Design review of the part built by this model. Coordinates are the model's own, in mm. A direction names the side the tool comes from. Coordinates: 2 decimals unless noted, no trailing zeros. Write each loop counter-clockwise with the first axis right and the second up, starting at its lowest first coordinate (ties: lowest second). Pieces come first, ordered by that corner, then holes. Notation, with made-up numbers: M 71,41.25 L 76,41.25 A21 cw 76,59.25 Z; hole C 17.25,41.25 d10. An arc over 180 degrees is marked long. One line per question, with ' | ' between items.
from build123d import *

# Parameters (mm, degrees)
F0_W     = 165.1
F0_H     = 44.45
F1_DEPTH = 88.9
F2_W     = 50.8
F2_H     = 12.7
F3_DEPTH = 165.1
F4_W     = 12.7
F4_H     = 12.7
F5_DEPTH = 165.1


with BuildPart() as f1:
    # F0 (on Front) → F1 (new body)
    with BuildSketch(Plane.XZ):
        with Locations((82.55, 22.225)):
            Rectangle(F0_W, F0_H)
    extrude(amount=F1_DEPTH)

    # F2 (on face) → F3 (cut)
    with BuildSketch(Plane.YZ.offset(165.1)):
        with Locations((-44.45, 6.35)):
            Rectangle(F2_W, F2_H)
    extrude(amount=-F3_DEPTH, mode=Mode.SUBTRACT)

    # F4 (on face) → F5 (cut)
    with BuildSketch(Plane.YZ.offset(165.1)):
        with Locations((-82.55, 38.1)):
            Rectangle(F4_W, F4_H)
        with Locations((-6.35, 38.1)):
            Rectangle(F4_W, F4_H)
    extrude(amount=-F5_DEPTH, mode=Mode.SUBTRACT)


solid = f1.part
1. Take a section at D-D (z = 35.5). Write out the cut boundary in (x, y).
Answer sheet:
outline: M 0,-76.2 L 165.1,-76.2 L 165.1,-12.7 L 0,-12.7 Z
2. Take a section at B-B (x = 116). Write out the cut boundary in (y, z), then the cut area to 3 significant figures.
Answer sheet:
outline: M -88.9,0 L -69.85,0 L -69.85,12.7 L -19.05,12.7 L -19.05,0 L 0,0 L 0,31.75 L -12.7,31.75 L -12.7,44.45 L -76.2,44.45 L -76.2,31.75 L -88.9,31.75 Z | area: 2,980 mm^2
3. Draft analysis for pull direction Y (two halves, no side actions). For faces 6 (the face through (84, -19.05, 6)), 7 (the face through (81, -79, 0)), 8 (the face through (84, -76.2, 38)), state which applies: pulls with the +Y half, pulls with the -Y half, needs draft (parallel to the pull), parting line crosses it, or undercut.
Answer sheet:
face 6: undercut | face 7: needs draft | face 8: pulls with the -Y half
4. To check wall thickness, follow line 1 along Y through (x, z) = (141, 7); line 2 along Z through (x, y) = (74.5, -66); line 3 along Z through (x, y) = (60.5, -79). State the ranges of each line that lie inside material, in increasing order. Write a range as [from, to].
Answer sheet:
line 1: [-88.9, -69.85], [-19.05, 0] | line 2: [12.7, 44.45] | line 3: [0, 31.75]
5. Take a section at A-A (z = 9.5). Write out the cut boundary in (x, y).
Answer sheet:
outline: M 0,-88.9 L 165.1,-88.9 L 165.1,-69.85 L 0,-69.85 Z; M 0,-19.05 L 165.1,-19.05 L 165.1,0 L 0,0 Z
6. Take a section at C-C (y = -79.5). Write out the cut boundary in (x, z).
Answer sheet:
outline: M 0,0 L 165.1,0 L 165.1,31.75 L 0,31.75 Z
7. Tool access review of faces 1 (the face through (84, -45, 12.7)), 2 (the face through (84, -83, 31.75)), 3 (the face through (84, -12.7, 38)), 4 (the face through (0, -44, 22)), 5 (the face through (81, -9, 0)): name each direction out of +Z, -Z, +X, -X, +Y, -Y from which nothing blocks a thin tool from reaching the whole face with its end or side.
Answer sheet:
face 1: -Z, +X, -X | face 2: +Z, +X, -X, -Y | face 3: +Z, +X, -X, +Y | face 4: +Z, -Z, -X, +Y, -Y | face 5: -Z, +X, -X, +Y, -Y
8. Insertion check: pin 1 Ø6.5 at (x, y) = (49, -84) entering from +Z; pin 2 Ø15 at (x, y) = (116, -50) entering from -Z; pin 3 Ø2 at (y, z) = (-40, 10) entering from -X; pin 4 Ø4 at (x, z) = (94, 35.5) entering from -Y. Each pin has a flat end and moves straight along its axis. Give the tip position at first contact, or say it passes through.
Answer sheet:
pin 1: z = 31.75 | pin 2: z = 12.7 | pin 3: through | pin 4: y = -76.2
